Answer from the drawing. Dimensions are ordinates in mm from the lowest x, y and z of the part. A direction names the side the tool comes from. Round coordinates to 2 decimals unless told otherwise and drop trailing zeros. Loops run counter-clockwise (first coordinate to the right, second up) from the corner with the lowest first, then second, coordinate; pieces in that order, holes last.
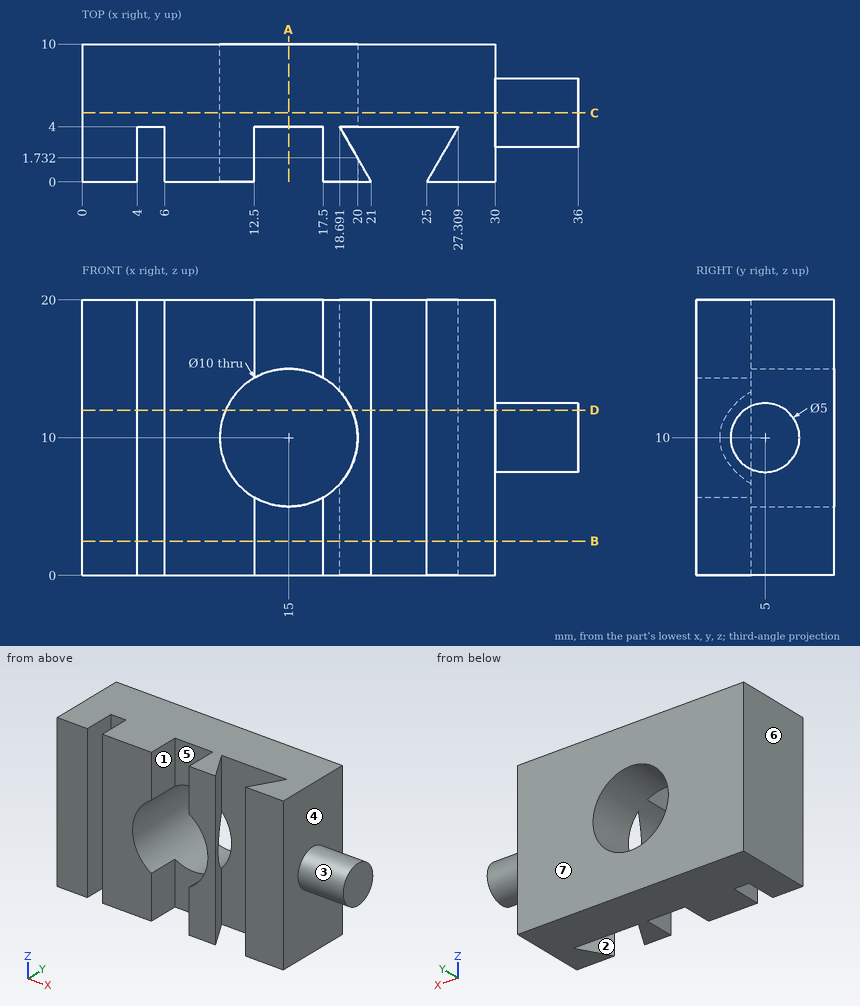
Item 1: Section A-A, the plane x = 15 is taken. Give the vertices of the cut face in (y, z).
Item 2: Section B-B, the plane z = 2.5 is taken. Give the vertices of the cut face in (x, y), plus the area to 3 significant figures.
Item 3: Straight lines are drawn through the part: line 1 (X direction, y = 1.75, z = 14); line 2 (Z direction, x = 15, y = 7); line 3 (X direction, y = 1, z = 14.75). For each, find the intervals that lie inside material, in ascending order.
Item 4: Section D-D, the plane z = 12 is taken. Give the vertices of the cut face in (x, y) (1 decimal), plus the area to 3 significant figures.
Item 5: Each of these flat-tipped pins is pushed along its axis until it touches: P1, Ø3, axis at y = 7, z = 5.5, coming from the +X side; P2, Ø2.5, axis at x = 15.5, z = 4, coming from the -Y side. Where does it stop, or does it pass through?
Item 6: Section C-C, the plane y = 5 is taken. Give the vertices of the cut face in (x, z).
Item 7: Determine the mould class of the marked faces 4, 5, 6 and 7 for opening direction X: pulls with the +X half, pulls with the -X half, needs draft (parallel to the pull), parting line crosses it, or undercut.
Item 8: For the marked faces 1, 2 and 3, determine the directions among +Z, -Z, +X, -X, +Y, -Y from which every point of the face is accessible in a straight line to the end or side of a thin tool.
Answer below:
1. outline: (4, 0) - (10, 0) - (10, 5) - (4, 5) - close; (4, 15) - (10, 15) - (10, 20) - (4, 20) - close
2. outline: (0, 0) - (4, 0) - (4, 4) - (6, 4) - (6, 0) - (12.5, 0) - (12.5, 4) - (17.5, 4) - (17.5, 0) - (21, 0) - (18.69, 4) - (27.31, 4) - (25, 0) - (30, 0) - (30, 10) - (0, 10) - close
2. area: 247 mm2
3. line 1: x = 0 to 4, 6 to 12, 18 to 19.99, 26.01 to 30
3. line 2: z = 0 to 5, 15 to 20
3. line 3: x = 0 to 4, 6 to 12.5, 17.5 to 20.42, 25.58 to 30
4. outline: (0, 0) - (4, 0) - (4, 4) - (6, 4) - (6, 0) - (10.4, 0) - (10.4, 10) - (0, 10) - close; (19.6, 0) - (21, 0) - (19.6, 2.5) - close; (19.6, 4) - (27.3, 4) - (25, 0) - (30, 0) - (30, 3.5) - (36, 3.5) - (36, 6.5) - (30, 6.5) - (30, 10) - (19.6, 10) - close
4. area: 194 mm2
5. P1: stops at x = 30
5. P2: stops at y = 4
6. outline: (0, 0) - (30, 0) - (30, 7.5) - (36, 7.5) - (36, 12.5) - (30, 12.5) - (30, 20) - (0, 20) - close; hole circle Ø10 at (15, 10)
7. face 4: pulls with the +X half
7. face 5: undercut
7. face 6: pulls with the -X half
7. face 7: needs draft
8. face 1: +Z, -Z, -Y
8. face 2: +Z, -Z
8. face 3: +X
